Could you check a few things on this model? Use its own coordinates, in mm. A direction names the side the tool comes from. Give positions to 0.01 mm unless a question says otherwise; leave off trailing zeros. Loops run counter-clockwise (first coordinate to the right, second up) from the corner with the lowest first, then second, coordinate; pieces in that order, holes last.
1. Imagine slicing it at A-A (x = 1.5). List the corners of the cut face in (y, z) for me, plus the area to 3 significant figures.
2. Imagine slicing it at C-C (y = 4.5). List the corners of the cut face in (x, z) for me.
3. For faces 1 (the cylindrical face through (-20, 10, 0)), 2 (the flat face through (25, 0, 4)), which set-ups out of +Z, -Z, +X, -X, +Y, -Y let a thin tool reach every point of the face, with its end or its side?
4. I need wall thicknesses on line 1 along Y through (x, z) = (10, -2.5); line 2 along Y through (x, z) = (25.5, -3); line 3 along X through (y, z) = (4, -12.5). Which ranges of each line are inside material? Lowest first, please.
5. Imagine slicing it at B-B (z = 15). List the corners of the cut face in (x, y) for me.
6. For P1, Ø5, axis at y = 23, z = -7.5, coming from the +X side; P2, Ø2, axis at y = 11, z = -4, coming from the -X side; P3, Ø24, axis at x = 29.5, z = 8, coming from the +Y side, each with a flat end and sliding along its axis, tell me the tip position at first contact or that it passes through.
7. Imagine slicing it at D-D (z = -4.5). List the corners of the cut face in (x, y) for me (3 decimals).
```python
from build123d import *

# Parameters (mm, degrees)
EXTRUDE_1_DEPTH = 10
EXTRUDE_START   = 30
EXTRUDE_2_DEPTH = 30
EXTRUDE_3_DEPTH = 20


with BuildPart() as part:
    # 草圖1 → 填料-伸長1 (new body)
    with BuildSketch(Plane(origin=(0, 0, 0), x_dir=(1, 0, 0), z_dir=(0, 1, 0))):
        with BuildLine():
            Line((0, -20), (40, -20))
            Line((40, -20), (30, 20))
            Line((30, 20), (0, 20))
            ThreePointArc((0, 20), (-20, 0), (0, -20))
        make_face()
    extrude(amount=-EXTRUDE_1_DEPTH)

    # 草圖2 → 填料-伸長2 (add)
    with BuildSketch(Plane(origin=(0, 0, 0), x_dir=(1, 0, 0), z_dir=(0, 1, 0)).offset(EXTRUDE_START)):
        with BuildLine():
            Line((10, 20), (0, 20))
            ThreePointArc((0, 20), (-20, 0), (0, -20))
            Line((0, -20), (10, 20))
        make_face()
    extrude(amount=-EXTRUDE_2_DEPTH)

    # 草圖2<3> → 填料-伸長3 (add)
    with BuildSketch(Plane(origin=(0, 0, 0), x_dir=(1, 0, 0), z_dir=(0, 1, 0))):
        Polygon((20.307764064, 20), (10, 20), (0, -20), (10.307764064, -20), align=None)
    extrude(amount=EXTRUDE_3_DEPTH)


solid = part.part
```
Derived:
1. outline: (-10, -20) - (30, -20) - (30, 14) - (20, 14) - (20, 20) - (-10, 20) - close
1. area: 1,540 mm2
2. outline: (0, -20) - (20.31, -20) - (10.31, 20) - (0, 20) arc R20 ccw to start
3. face 1: -X, +Y, -Y
3. face 2: +Z, +X, +Y
4. line 1: y = -10 to 20
4. line 2: y = -10 to 0
4. line 3: x = -15.61 to 18.43
5. outline: (-13.23, -10) - (38.75, -10) - (38.75, 0) - (11.56, 0) - (11.56, 20) - (1.25, 20) - (1.25, 30) - (-13.23, 30) - close
6. P1: stops at x = 7.5
6. P2: stops at x = -19.77
6. P3: stops at y = 0
7. outline: (-19.487, -10) - (33.875, -10) - (33.875, 0) - (16.433, 0) - (16.433, 20) - (6.125, 20) - (6.125, 30) - (-19.487, 30) - close
